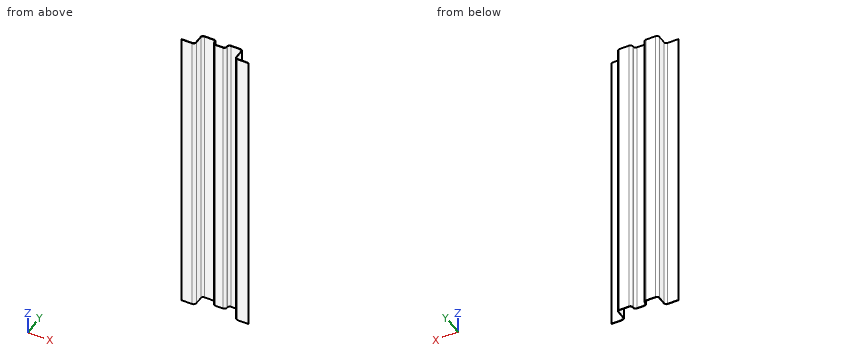
Autodesk Inventor part; units mm, degrees
ref_plane "YZ Plane" through (0, 0, 0) normal (1, 0, 0) x (0, 1, 0)
ref_plane "XZ Plane" through (0, 0, 0) normal (0, 1, 0) x (-1, 0, 0)
ref_plane "XY Plane" through (0, 0, 0) normal (0, 0, 1) x (1, 0, 0)
sketch "Sketch1" plane through (0, 0, 0) normal (0, 0, 1) x (1, 0, 0)
  line L0 (-41.8, 0) -> (-61.75, 0)
  line L1 (-15.75, 24.3) -> (-33, 24.3)
  line L2 (0, 14.3) -> (-6.95, 14.3)
  line L3 (-11.75, 20.3) -> (-11.75, 19.1)
  line L4 (-37, 20.3) -> (-37, 4.8)
  arc A0 (-11.75, 19.1) -> (-6.95, 14.3) centre (-6.95, 19.1) ccw
  arc A1 (-11.75, 20.3) -> (-15.75, 24.3) centre (-15.75, 20.3) ccw
  arc A2 (-33, 24.3) -> (-37, 20.3) centre (-33, 20.3) ccw
  arc A3 (-41.8, 0) -> (-37, 4.8) centre (-41.8, 4.8) ccw
  line L5 (-61.75, 0.8) -> (-41.8, 0.8)
  arc A4 (-41.8, 0.8) -> (-37.8, 4.8) centre (-41.8, 4.8) ccw
  line L6 (-37.8, 4.8) -> (-37.8, 20.3)
  arc A5 (-33, 25.1) -> (-37.8, 20.3) centre (-33, 20.3) ccw
  line L7 (-33, 25.1) -> (-15.75, 25.1)
  arc A6 (-10.95, 20.3) -> (-15.75, 25.1) centre (-15.75, 20.3) ccw
  line L8 (-10.95, 20.3) -> (-10.95, 19.1)
  arc A7 (-10.95, 19.1) -> (-6.95, 15.1) centre (-6.95, 19.1) ccw
  line L9 (-6.95, 15.1) -> (0, 15.1)
  line L10 (-61.75, 0) -> (-61.75, 0.8)
  line L11 (0, 0) -> (0, 9.3563)
  line L12 (0, 14.3) -> (0, 15.1)
  dimension "d0" = 14.3
  dimension "d2" = 24.3
  dimension "d4" = 25.25
  dimension "d5" = 4.8
  dimension "d6" = 4
  dimension "d8" = 0.8
  dimension "d11" = 6.95
  dimension "d12" = 19.95
extrude "Extrusion1" add sketch "Sketch1" along normal mid plane 545
mirror "Mirror1" about plane through (0, 0, 0) normal (1, 0, 0) of "Extrusion1"
properties part number "AAD0001106802"
CAD build for the part. Positions are in the model's coordinates, mm. Give positions to 0.01 mm unless a question says otherwise; leave off trailing zeros. Write each loop counter-clockwise with the first axis right and the second up, starting at its lowest first coordinate (ties: lowest second). Pieces come first, ordered by that corner, then holes. Notation, with made-up numbers: M 78.5,-8 L 124.5,-8 A21 cw 124.5,19 Z; hole C 13.25,72.25 d5. An arc over 180 degrees is marked long. Return JSON: item names as keys, results as strings. Group by question number.
(1) Drill centre lines: L1, parallel to X at y = 12.5, z = -28; L2, parallel to X at y = 17.5, z = 94.5; L3, parallel to Y at x = -42.5, z = 180.5. Where is each one in solid material? Low to high. Write a range as [from, to].
(2) Band-saw the part on A-A (x = -27). Give the cut face in (y, z), and give its area (3 significant figures).
(3) Flat gauge pins, fed straight in: pin 1 Ø19 at (x, z) = (27, 35.5) entering from -Y; pin 2 Ø11 at (x, z) = (2.5, 57.5) entering from +Y; pin 3 Ø5 at (x, z) = (-24, -121) entering from -Y. Where does each tip first touch, or does it go through?
Entries:
{
 "1": {"L1": "x = [-37.8, -37], [37, 37.8]", "L2": "x = [-37.8, -37], [-11.48, -10.62], [10.62, 11.48], [37, 37.8]", "L3": "y = [0, 0.8]"},
 "2": {"outline": "M 24.3,-272.5 L 25.1,-272.5 L 25.1,272.5 L 24.3,272.5 Z", "area": "436 mm^2"},
 "3": {"pin 1": "stops at y = 22.24", "pin 2": "stops at y = 15.24", "pin 3": "stops at y = 24.3"}
}
